Source: CAD feature listing. Evaluate the final solid. Frame: model axes, mm. Coordinates: 2 decimals unless noted, no trailing zeros. Order: outer loops, then holes, each group sorted by start corner. A loop starts at its lowest first (then second) coordinate and runs counter-clockwise, first axis right, second up.
```python
from build123d import *

# Parameters (mm, degrees)
F0_R     = 12.7
F1_DEPTH = 12.7


with BuildPart() as f1:
    # F0 (on Front) → F1 (new body, symmetric)
    with BuildSketch(Plane.XZ):
        with BuildLine():
            ThreePointArc((0, 6.35), (1.859872, 1.859872), (6.35, 0))
            Line((6.35, 0), (64.526166, 0))
            ThreePointArc((64.526166, 0), (69.016294, 1.859872), (70.876166, 6.35))
            Line((70.876166, 6.35), (70.876166, 53.155664))
            ThreePointArc((70.876166, 53.155664), (69.016294, 57.645792), (64.526166, 59.505664))
            Line((64.526166, 59.505664), (6.35, 59.505664))
            ThreePointArc((6.35, 59.505664), (1.859872, 57.645792), (0, 53.155664))
            Line((0, 53.155664), (0, 6.35))
        make_face()
        with Locations((35.627604, 31.458408)):
            Circle(F0_R, mode=Mode.SUBTRACT)
    extrude(amount=F1_DEPTH, both=True)


solid = f1.part
```
1. Material intervals for line 1 along X through (y, z) = (-2, 33.5); line 2 along Z through (x, y) = (31, -2.25); line 3 along Z through (x, y) = (47, -10.25), sorted ascending.
2. Section query B-B, the plane z = 35. Output: boundary loops of the cut face in (x, y).
3. Section query A-A, the plane x = 44.5. Output: boundary loops of the cut face in (y, z).
4. Section query C-C, the plane y = 5.25. Output: boundary loops of the cut face in (x, z).
5. Draft query along X for faces 1 (the cylindrical face through (69.065, -0.178, 57.596)), 2 (the flat face through (36, 0, 59.506)), 3 (the cylindrical face through (33.97, 0.18, 44.05)). Return one class per face: +X half, -X half, draft (parallel to the pull), parting line (faces both ways), or undercut.
Answer key:
1. line 1: x = 0 to 23.09, 48.16 to 70.88
1. line 2: z = 0 to 19.63, 43.29 to 59.51
1. line 3: z = 0 to 25.81, 37.11 to 59.51
2. outline: (0, -12.7) - (23.43, -12.7) - (23.43, 12.7) - (0, 12.7) - close; (47.82, -12.7) - (70.88, -12.7) - (70.88, 12.7) - (47.82, 12.7) - close
3. outline: (-12.7, 0) - (12.7, 0) - (12.7, 22.37) - (-12.7, 22.37) - close; (-12.7, 40.55) - (12.7, 40.55) - (12.7, 59.51) - (-12.7, 59.51) - close
4. outline: (0, 6.35) arc R6.35 ccw to (6.35, 0) - (64.53, 0) arc R6.35 ccw to (70.88, 6.35) - (70.88, 53.16) arc R6.35 ccw to (64.53, 59.51) - (6.35, 59.51) arc R6.35 ccw to (0, 53.16) - close; hole circle Ø25.4 at (35.63, 31.46)
5. face 1: +X half
5. face 2: draft
5. face 3: undercut
